Model file for the job. Use its own axes, mm. A direction names the side the tool comes from. Give positions to 0.01 mm unless a question says otherwise; leave off trailing zeros. Loops run counter-clockwise (first coordinate to the right, second up) from the corner with the lowest first, then second, coordinate; pieces in that order, holes last. Notation, with made-up numbers: M -15,55.25 L 3,55.25 A27 cw 3,71.25 Z; hole C -34,43.25 d1. An arc over 180 degrees is marked long. Answer in a Markdown table with one row per item.
```python
from build123d import *

# Parameters (mm, degrees)
SKETCH_R        = 7.5
SKETCH_R_2      = 5.5
PAD_DEPTH       = 2
SKETCH001_R     = 7
SKETCH001_R_2   = 3.5
PAD001_DEPTH    = 4
SKETCH002_R     = 5
PAD002_DEPTH    = 9
SKETCH003_W     = 10.5
SKETCH003_H     = 4
PAD003_DEPTH    = 4
SKETCH004_R     = 1.15
POCKET_DEPTH    = 12.751
SKETCH005_R     = 9
POCKET001_DEPTH = 9
SKETCH006_W     = 1.5
SKETCH006_H     = 9
POCKET002_DEPTH = 15.001
SKETCH007_W     = 3
SKETCH007_H     = 9
POCKET003_DEPTH = 5
SKETCH008_W     = 15
SKETCH008_H     = 8
PAD004_DEPTH    = 7.5
POCKET004_DEPTH = 6.3


with BuildPart() as part:
    # Sketch → Pad (new body)
    with BuildSketch(Plane.XY):
        Circle(SKETCH_R)
        Circle(SKETCH_R_2, mode=Mode.SUBTRACT)
    extrude(amount=PAD_DEPTH)

    # Sketch001 (on Face4 of Pad) → Pad001 (join)
    with BuildSketch(Plane.XY.offset(2)):
        Circle(SKETCH001_R)
        Circle(SKETCH001_R_2, mode=Mode.SUBTRACT)
    extrude(amount=PAD001_DEPTH)

    # Sketch002 (on Face7 of Pad001) → Pad002 (join)
    with BuildSketch(Plane.XY.offset(6)):
        Circle(SKETCH002_R)
        with BuildLine():
            ThreePointArc((1.75, 0.85), (0, 2.6), (-1.75, 0.85))
            Line((-1.75, 0.85), (-1.75, -0.85))
            ThreePointArc((-1.75, -0.85), (0, -2.6), (1.75, -0.85))
            Line((1.75, 0.85), (1.75, -0.85))
        make_face(mode=Mode.SUBTRACT)
    extrude(amount=PAD002_DEPTH)

    # Sketch003 (on Face3 of Pad002) → Pad003 (join)
    with BuildSketch(Plane.XY.offset(2)):
        with Locations((0, 6)):
            Rectangle(SKETCH003_W, SKETCH003_H)
    extrude(amount=PAD003_DEPTH)

    # Sketch004 (on Face6 of Pad003) → Pocket (cut, through all)
    with BuildSketch(Plane(origin=(-5.25, 0, 0), x_dir=(0, -1, 0), z_dir=(-1, 0, 0))):
        with Locations((-6, 4)):
            Circle(SKETCH004_R)
    extrude(amount=-POCKET_DEPTH, mode=Mode.SUBTRACT)

    # Sketch005 (on Face20 of Pocket) → Pocket001 (cut)
    with BuildSketch(Plane.XY.offset(15)):
        Circle(SKETCH005_R)
        Polygon((0.5, 8.5), (0, 3), (-0.5, 8.5), (-8.5, 2), (-2.5, 0), (-8.5, -2), (-0.5, -8.5), (0, -3), (0.5, -8.5), (8.5, -2), (2.5, 0), (8.5, 2), align=None, mode=Mode.SUBTRACT)
    extrude(amount=-POCKET001_DEPTH, mode=Mode.SUBTRACT)

    # Sketch006 (on Face2 of Pocket001) → Pocket002 (cut, through all)
    with BuildSketch(Plane(origin=(0, 0, 0), x_dir=(1, 0, 0), z_dir=(0, 0, -1))):
        with Locations((0, -4.5)):
            Rectangle(SKETCH006_W, SKETCH006_H)
    extrude(amount=-POCKET002_DEPTH, mode=Mode.SUBTRACT)

    # Sketch007 (on Face16 of Pocket002) → Pocket003 (cut)
    with BuildSketch(Plane(origin=(0, 0, 2), x_dir=(1, 0, 0), z_dir=(0, 0, -1))):
        with Locations((0, 4.5)):
            Rectangle(SKETCH007_W, SKETCH007_H)
    extrude(amount=-POCKET003_DEPTH, mode=Mode.SUBTRACT)

    # Sketch008 (on Face24 of Pocket003) → Pad004 (join, symmetric)
    with BuildSketch(Plane.XY.offset(15)):
        with Locations((0, -7)):
            Rectangle(SKETCH008_W, SKETCH008_H)
    extrude(amount=PAD004_DEPTH, both=True)

    # Sketch009 (on Face78 of Pad004) → Pocket004 (cut)
    with BuildSketch(Plane.XZ.offset(11)):
        Polygon((0, 21.408588), (-5.55, 18.204294), (-5.55, 11.795706), (0, 8.591412), (5.55, 11.795706), (5.55, 18.204294), align=None)
    extrude(amount=-POCKET004_DEPTH, mode=Mode.SUBTRACT)


solid = part.part
```
Q1. Probe probe 1 along X at (y, z) = (0, 1.45); probe 2 along Y at (x, z) = (4.5, 11.5); probe 3 along Z at (x, y) = (-3.5, 6). List the from-to ranges inside material, lowest first.
Reported:
| item | result |
|---|---|
| probe 1 | -7.5 to -5.5, 5.5 to 7.5 |
| probe 2 | -4.7 to -3, -2.18 to -0.67, 0.67 to 2.18 |
| probe 3 | 0 to 2.85, 5.15 to 6 |
Q2. Saw through at D-D (z = 14.5). Give the cut face in (x, y), and give its area (3 significant figures).
Reported:
| item | result |
|---|---|
| outline | M -7.5,-11 L -5.55,-11 L -5.55,-4.7 L 5.55,-4.7 L 5.55,-11 L 7.5,-11 L 7.5,-3 L 4,-3 A5 ccw 4.93,-0.81 L 2.5,0 L 4.93,0.81 A5 ccw 0.75,4.94 L 0.75,2.43 A1.75 cw 1.75,0.85 L 1.75,-0.85 A1.75 cw -1.75,-0.85 L -1.75,0.85 A1.75 cw -0.75,2.43 L -0.75,4.94 A5 ccw -4.93,0.81 L -2.5,0 L -4.93,-0.81 A5 ccw -4,-3 L -7.5,-3 Z |
| area | 94.1 mm² |
Q3. Saw through at C-C (y = 6). Give the cut face in (x, z).
Reported:
| item | result |
|---|---|
| outline | M -5.25,2 L -4.5,2 L -4.5,0 L -0.75,0 L -0.75,2.85 L -5.25,2.85 Z; M -5.25,5.15 L -0.75,5.15 L -0.75,6 L -5.25,6 Z; M 0.75,0 L 4.5,0 L 4.5,2 L 5.25,2 L 5.25,2.85 L 0.75,2.85 Z; M 0.75,5.15 L 5.25,5.15 L 5.25,6 L 0.75,6 Z |
Q4. 3-axis set-ups, long thin cutter, end or side, ignore diameter. For faces 1 (the face through (1.49, 1.77, 10.44)), 2 (the face through (-3.47, 0.46, 3.97)), 3 (the face through (-2.736, -7.894, 19.829)), 4 (the face through (-3, 4, 10)): which of +Z, -Z, +X, -X, +Y, -Y reach the whole face in a straight line?
Reported:
| item | result |
|---|---|
| face 1 | +Z, -Z |
| face 2 | -Z |
| face 3 | -Y |
| face 4 | +Z, -X, +Y |
Q5. Drop flat-ended pins along their axis: pin 1 (2.5 mm diameter, centred on x = -2, y = -2.5, fed in from -Z); pin 2 (2.5 mm diameter, centred on y = -4, z = 5.5, fed in from +X); pin 3 (3.5 mm diameter, centred on x = -2, z = 13.5, fed in from -Y). Give the stop position or say it passes through.
Reported:
| item | result |
|---|---|
| pin 1 | z = 2 |
| pin 2 | x = 6.44 |
| pin 3 | y = -4.7 |
Q6. Mould opens along Y. For faces 5 (the face through (-2, 0, 6)), 6 (the face through (-3, 8, 4)), 7 (the face through (-4, 0, 2)), 8 (the face through (0, -7, 22.5)) say: released by +Y, released by -Y, zero draft, split by the parting line, or undercut.
Reported:
| item | result |
|---|---|
| face 5 | undercut |
| face 6 | released by +Y |
| face 7 | undercut |
| face 8 | zero draft |
Q7. Saw through at B-B (y = -8.25). Give the cut face in (x, z).
Reported:
| item | result |
|---|---|
| outline | M -7.5,7.5 L 7.5,7.5 L 7.5,22.5 L -7.5,22.5 Z; hole M -5.55,11.8 L 0,8.59 L 5.55,11.8 L 5.55,18.2 L 0,21.41 L -5.55,18.2 Z |
Q8. Saw through at A-A (z = 4). Give the cut face in (x, y).
Reported:
| item | result |
|---|---|
| outline | M -5.25,4.63 A7 ccw -1.5,-6.84 L -1.5,-3.16 A3.5 cw -0.75,3.42 L -0.75,4.85 L -5.25,4.85 Z; M -5.25,7.15 L -0.75,7.15 L -0.75,8 L -5.25,8 Z; M 0.75,3.42 A3.5 cw 1.5,-3.16 L 1.5,-6.84 A7 ccw 5.25,4.63 L 5.25,4.85 L 0.75,4.85 Z; M 0.75,7.15 L 5.25,7.15 L 5.25,8 L 0.75,8 Z |
